```python
from build123d import *

# Parameters (mm, degrees)
F0_R     = 4.35
F1_DEPTH = 2.35
F2_DEPTH = 1
F3_DEPTH = 25


# Not quite as in the source:
# - a feature names something its author has since deleted; it is built from what else it names


with BuildPart() as f1:
    # F0 (on Front) → F1 (new body)
    with BuildSketch(Plane.XZ):
        with BuildLine():
            ThreePointArc((18.9519787885, 1.35), (18.9879909019, 0.6754269088), (19, 0))
            ThreePointArc((19, 0), (18.9879909019, -0.6754269088), (18.9519787885, -1.35))
            ThreePointArc((18.9519787885, -1.35), (13.4350288425, -13.4350288425), (1.35, -18.9519787885))
            ThreePointArc((1.35, -18.9519787885), (0, -19), (-1.35, -18.9519787885))
            ThreePointArc((-1.35, -18.9519787885), (-13.4350288425, -13.4350288425), (-18.9519787885, -1.35))
            ThreePointArc((-18.9519787885, -1.35), (-19, 0), (-18.9519787885, 1.35))
            ThreePointArc((-18.9519787885, 1.35), (-18.0084373125, 6.0577376603), (-15.9148967645, 10.378634832))
            ThreePointArc((-15.9148967645, 10.378634832), (-16.5717114004, 10.7446905008), (-17.1694954771, 11.2008225173))
            ThreePointArc((-17.1694954771, 11.2008225173), (-19.4465872664, 6.4869286792), (-20.4555004828, 1.35))
            ThreePointArc((-20.4555004828, 1.35), (-20.5, 0), (-20.4555004828, -1.35))
            ThreePointArc((-20.4555004828, -1.35), (-14.4956890143, -14.4956890143), (-1.35, -20.4555004828))
            ThreePointArc((-1.35, -20.4555004828), (0, -20.5), (1.35, -20.4555004828))
            ThreePointArc((1.35, -20.4555004828), (14.4956890143, -14.4956890143), (20.4555004828, -1.35))
            ThreePointArc((20.4555004828, -1.35), (20.4888721004, -0.6753666055), (20.5, 0))
            ThreePointArc((20.5, 0), (20.4888721004, 0.6753666055), (20.4555004828, 1.35))
            ThreePointArc((20.4555004828, 1.35), (14.4956890143, 14.4956890143), (1.35, 20.4555004828))
            ThreePointArc((1.35, 20.4555004828), (0, 20.5), (-1.35, 20.4555004828))
            ThreePointArc((-1.35, 20.4555004828), (-5.5075668443, 19.7463087046), (-9.4320097524, 18.2012964382))
            ThreePointArc((-9.4320097524, 18.2012964382), (-9.0377919084, 17.5609883013), (-8.7390902551, 16.8709306653))
            ThreePointArc((-8.7390902551, 16.8709306653), (-5.1507403222, 18.2885175488), (-1.35, 18.9519787885))
            ThreePointArc((-1.35, 18.9519787885), (0, 19), (1.35, 18.9519787885))
            ThreePointArc((1.35, 18.9519787885), (13.4350288425, 13.4350288425), (18.9519787885, 1.35))
        make_face()
        with BuildLine():
            ThreePointArc((-1.35, -18.9519787885), (0, -19), (1.35, -18.9519787885))
            Line((1.35, -18.9519787885), (1.35, -5.7948252778))
            ThreePointArc((1.35, -5.7948252778), (0, -5.95), (-1.35, -5.7948252778))
            Line((-1.35, -5.7948252778), (-1.35, -18.9519787885))
        make_face()
        with BuildLine():
            ThreePointArc((18.9519787885, -1.35), (18.9879909019, -0.6754269088), (19, 0))
            ThreePointArc((19, 0), (18.9879909019, 0.6754269088), (18.9519787885, 1.35))
            Line((18.9519787885, 1.35), (5.7948252778, 1.35))
            ThreePointArc((5.7948252778, 1.35), (5.9110790218, 0.6794444779), (5.95, 0))
            ThreePointArc((5.95, 0), (5.9110790218, -0.6794444779), (5.7948252778, -1.35))
            Line((5.7948252778, -1.35), (18.9519787885, -1.35))
        make_face()
        with BuildLine():
            ThreePointArc((-18.9519787885, 1.35), (-19, 0), (-18.9519787885, -1.35))
            Line((-18.9519787885, -1.35), (-5.7948252778, -1.35))
            ThreePointArc((-5.7948252778, -1.35), (-5.95, 0), (-5.7948252778, 1.35))
            Line((-5.7948252778, 1.35), (-18.9519787885, 1.35))
        make_face()
        with BuildLine():
            Line((1.35, 5.7948252778), (1.35, 18.9519787885))
            ThreePointArc((1.35, 18.9519787885), (0, 19), (-1.35, 18.9519787885))
            Line((-1.35, 18.9519787885), (-1.35, 5.7948252778))
            ThreePointArc((-1.35, 5.7948252778), (0, 5.95), (1.35, 5.7948252778))
        make_face()
        with BuildLine():
            ThreePointArc((5.95, 0), (5.9110790218, 0.6794444779), (5.7948252778, 1.35))
            ThreePointArc((5.7948252778, 1.35), (4.2072853481, 4.2072853481), (1.35, 5.7948252778))
            ThreePointArc((1.35, 5.7948252778), (0, 5.95), (-1.35, 5.7948252778))
            ThreePointArc((-1.35, 5.7948252778), (-4.2072853481, 4.2072853481), (-5.7948252778, 1.35))
            ThreePointArc((-5.7948252778, 1.35), (-5.95, 0), (-5.7948252778, -1.35))
            ThreePointArc((-5.7948252778, -1.35), (-4.2072853481, -4.2072853481), (-1.35, -5.7948252778))
            ThreePointArc((-1.35, -5.7948252778), (0, -5.95), (1.35, -5.7948252778))
            ThreePointArc((1.35, -5.7948252778), (4.2072853481, -4.2072853481), (5.7948252778, -1.35))
            ThreePointArc((5.7948252778, -1.35), (5.9110790218, -0.6794444779), (5.95, 0))
        make_face()
        Circle(F0_R, mode=Mode.SUBTRACT)
    extrude(amount=F1_DEPTH)

    # F0 (on Front) → F2 (join)
    with BuildSketch(Plane.XZ):
        with BuildLine():
            Line((-1.35, 5.7948252778), (-1.35, 18.9519787885))
            ThreePointArc((-1.35, 18.9519787885), (-5.1507403222, 18.2885175488), (-8.7390902551, 16.8709306653))
            ThreePointArc((-8.7390902551, 16.8709306653), (-10.1717962693, 11.2426857548), (-15.9148967645, 10.378634832))
            ThreePointArc((-15.9148967645, 10.378634832), (-18.0084373125, 6.0577376603), (-18.9519787885, 1.35))
            Line((-18.9519787885, 1.35), (-5.7948252778, 1.35))
            ThreePointArc((-5.7948252778, 1.35), (-4.2072853481, 4.2072853481), (-1.35, 5.7948252778))
        make_face()
        with BuildLine():
            ThreePointArc((1.35, -18.9519787885), (13.4350288425, -13.4350288425), (18.9519787885, -1.35))
            Line((18.9519787885, -1.35), (5.7948252778, -1.35))
            ThreePointArc((5.7948252778, -1.35), (4.2072853481, -4.2072853481), (1.35, -5.7948252778))
            Line((1.35, -5.7948252778), (1.35, -18.9519787885))
        make_face()
        with BuildLine():
            Line((5.7948252778, 1.35), (18.9519787885, 1.35))
            ThreePointArc((18.9519787885, 1.35), (13.4350288425, 13.4350288425), (1.35, 18.9519787885))
            Line((1.35, 18.9519787885), (1.35, 5.7948252778))
            ThreePointArc((1.35, 5.7948252778), (4.2072853481, 4.2072853481), (5.7948252778, 1.35))
        make_face()
        with BuildLine():
            ThreePointArc((-18.9519787885, -1.35), (-13.4350288425, -13.4350288425), (-1.35, -18.9519787885))
            Line((-1.35, -18.9519787885), (-1.35, -5.7948252778))
            ThreePointArc((-1.35, -5.7948252778), (-4.2072853481, -4.2072853481), (-5.7948252778, -1.35))
            Line((-5.7948252778, -1.35), (-18.9519787885, -1.35))
        make_face()
        with BuildLine():
            ThreePointArc((-20.4555004828, -1.35), (-20.5, 0), (-20.4555004828, 1.35))
            ThreePointArc((-20.4555004828, 1.35), (-21.8055004828, 0), (-20.4555004828, -1.35))
        make_face()
        with BuildLine():
            ThreePointArc((1.35, -20.4555004828), (0, -20.5), (-1.35, -20.4555004828))
            ThreePointArc((-1.35, -20.4555004828), (0, -21.8055004828), (1.35, -20.4555004828))
        make_face()
        with BuildLine():
            ThreePointArc((20.4555004828, -1.35), (21.8055004828, 0), (20.4555004828, 1.35))
            ThreePointArc((20.4555004828, 1.35), (20.4888721004, 0.6753666055), (20.5, 0))
            ThreePointArc((20.5, 0), (20.4888721004, -0.6753666055), (20.4555004828, -1.35))
        make_face()
        with BuildLine():
            ThreePointArc((1.35, 20.4555004828), (0, 21.8055004828), (-1.35, 20.4555004828))
            ThreePointArc((-1.35, 20.4555004828), (0, 20.5), (1.35, 20.4555004828))
        make_face()
    extrude(amount=F2_DEPTH)

    # F0 (on Front) → F3 (cut)
    with BuildSketch(Plane.XZ):
        with BuildLine():
            ThreePointArc((18.9519787885, 1.35), (18.9879909019, 0.6754269088), (19, 0))
            ThreePointArc((19, 0), (18.9879909019, -0.6754269088), (18.9519787885, -1.35))
            ThreePointArc((18.9519787885, -1.35), (13.4350288425, -13.4350288425), (1.35, -18.9519787885))
            ThreePointArc((1.35, -18.9519787885), (0, -19), (-1.35, -18.9519787885))
            ThreePointArc((-1.35, -18.9519787885), (-13.4350288425, -13.4350288425), (-18.9519787885, -1.35))
            ThreePointArc((-18.9519787885, -1.35), (-19, 0), (-18.9519787885, 1.35))
            ThreePointArc((-18.9519787885, 1.35), (-18.0084373125, 6.0577376603), (-15.9148967645, 10.378634832))
            ThreePointArc((-15.9148967645, 10.378634832), (-16.5717114004, 10.7446905008), (-17.1694954771, 11.2008225173))
            ThreePointArc((-17.1694954771, 11.2008225173), (-19.4465872664, 6.4869286792), (-20.4555004828, 1.35))
            ThreePointArc((-20.4555004828, 1.35), (-20.5, 0), (-20.4555004828, -1.35))
            ThreePointArc((-20.4555004828, -1.35), (-14.4956890143, -14.4956890143), (-1.35, -20.4555004828))
            ThreePointArc((-1.35, -20.4555004828), (0, -20.5), (1.35, -20.4555004828))
            ThreePointArc((1.35, -20.4555004828), (14.4956890143, -14.4956890143), (20.4555004828, -1.35))
            ThreePointArc((20.4555004828, -1.35), (20.4888721004, -0.6753666055), (20.5, 0))
            ThreePointArc((20.5, 0), (20.4888721004, 0.6753666055), (20.4555004828, 1.35))
            ThreePointArc((20.4555004828, 1.35), (14.4956890143, 14.4956890143), (1.35, 20.4555004828))
            ThreePointArc((1.35, 20.4555004828), (0, 20.5), (-1.35, 20.4555004828))
            ThreePointArc((-1.35, 20.4555004828), (-5.5075668443, 19.7463087046), (-9.4320097524, 18.2012964382))
            ThreePointArc((-9.4320097524, 18.2012964382), (-9.0377919084, 17.5609883013), (-8.7390902551, 16.8709306653))
            ThreePointArc((-8.7390902551, 16.8709306653), (-5.1507403222, 18.2885175488), (-1.35, 18.9519787885))
            ThreePointArc((-1.35, 18.9519787885), (0, 19), (1.35, 18.9519787885))
            ThreePointArc((1.35, 18.9519787885), (13.4350288425, 13.4350288425), (18.9519787885, 1.35))
        make_face()
        with BuildLine():
            ThreePointArc((-15.9148967645, 10.378634832), (-12.7472446155, 14.0892780054), (-8.7390902551, 16.8709306653))
            ThreePointArc((-8.7390902551, 16.8709306653), (-9.0377919084, 17.5609883013), (-9.4320097524, 18.2012964382))
            ThreePointArc((-9.4320097524, 18.2012964382), (-13.7536060325, 15.2015894268), (-17.1694954771, 11.2008225173))
            ThreePointArc((-17.1694954771, 11.2008225173), (-16.5717114004, 10.7446905008), (-15.9148967645, 10.378634832))
        make_face()
        with BuildLine():
            ThreePointArc((1.35, 20.4555004828), (0, 21.8055004828), (-1.35, 20.4555004828))
            ThreePointArc((-1.35, 20.4555004828), (0, 20.5), (1.35, 20.4555004828))
        make_face()
        with BuildLine():
            ThreePointArc((-20.4555004828, -1.35), (-20.5, 0), (-20.4555004828, 1.35))
            ThreePointArc((-20.4555004828, 1.35), (-21.8055004828, 0), (-20.4555004828, -1.35))
        make_face()
        with BuildLine():
            ThreePointArc((20.4555004828, -1.35), (21.8055004828, 0), (20.4555004828, 1.35))
            ThreePointArc((20.4555004828, 1.35), (20.4888721004, 0.6753666055), (20.5, 0))
            ThreePointArc((20.5, 0), (20.4888721004, -0.6753666055), (20.4555004828, -1.35))
        make_face()
        with BuildLine():
            ThreePointArc((1.35, -20.4555004828), (0, -20.5), (-1.35, -20.4555004828))
            ThreePointArc((-1.35, -20.4555004828), (0, -21.8055004828), (1.35, -20.4555004828))
        make_face()
    extrude(amount=-F3_DEPTH, mode=Mode.SUBTRACT)


solid = f1.part
```
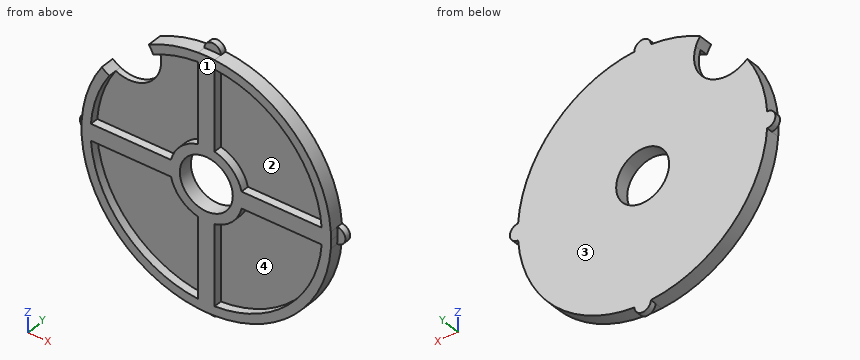
Model file for the job. Use its own axes, mm. Face numbers are marked on the shaded views. A direction names the side the tool comes from. Give positions to 0.01 mm unless a question says otherwise; leave off trailing zeros. Order: outer loops, then holes, each group sorted by start corner. A loop starts at its lowest first (then second) coordinate and runs counter-clockwise, first axis right, second up.
1) Saw through at B-B, the plane y = -0.45. Write the cut outline in (x, z).
2) 3-axis set-ups, long thin cutter, end or side, ignore diameter. For the marked faces 3 and 4: which of +Z, -Z, +X, -X, +Y, -Y reach the whole face in a straight line?
3) Mould opens along Z. For the marked faces 1 and 2 say: +Z half, -Z half, draft (parallel to the pull), parting line (faces both ways), or undercut.
4) Saw through at C-C, the plane z = -3. Write the cut outline in (x, y), then the cut area to 3 significant figures.
5) Saw through at D-D, the plane x = 13. Write the cut outline in (y, z), then the cut area to 3 significant figures.
6) Wall check: probe 1 along Z at (x, y) = (0, -1.55); probe 2 along Z at (x, y) = (0, -0.85); probe 3 along Z at (x, y) = (-7.5, -1.05). Give the ranges that are in metal, low to high.
7) Saw through at A-A, the plane x = 0. Write the cut outline in (y, z).
8) Pin check, flat tips, straight feed: pin 1 (5 mm diameter, centred on x = 6, z = -10.5, fed in from +Y); pin 2 (1 mm diameter, centred on y = -1, z = -7.5, fed in from -X); pin 3 (1.1 mm diameter, centred on x = -11.5, y = -1.5, fed in from -Z); pin 4 (1.1 mm diameter, centred on x = 9.5, y = -1.5, fed in from +Z). Stop position of each tip, or through.
Computed:
1. outline: (-20.46, -1.35) arc R20.5 ccw to (-1.35, -20.46) arc R1.35 ccw to (1.35, -20.46) arc R20.5 ccw to (20.46, -1.35) arc R1.35 ccw to (20.46, 1.35) arc R20.5 ccw to (1.35, 20.46) arc R1.35 ccw to (-1.35, 20.46) arc R20.5 ccw to (-9.43, 18.2) arc R5.25 cw to (-17.17, 11.2) arc R20.5 ccw to (-20.46, 1.35) arc R1.35 ccw to start; hole circle Ø8.7 at (0, 0)
2. face 3: +Z, -Z, +X, -X, +Y
2. face 4: -Y
3. face 1: draft
3. face 2: undercut
4. outline: (-20.28, -2.35) - (-18.76, -2.35) - (-18.76, -1) - (-5.14, -1) - (-5.14, -2.35) - (-3.15, -2.35) - (-3.15, 0) - (-20.28, 0) - close; (3.15, -2.35) - (5.14, -2.35) - (5.14, -1) - (18.76, -1) - (18.76, -2.35) - (20.28, -2.35) - (20.28, 0) - (3.15, 0) - close
4. area: 43.7 mm2
5. outline: (-2.35, -15.85) - (0, -15.85) - (0, 15.85) - (-2.35, 15.85) - (-2.35, 13.86) - (-1, 13.86) - (-1, 1.35) - (-2.35, 1.35) - (-2.35, -1.35) - (-1, -1.35) - (-1, -13.86) - (-2.35, -13.86) - close
5. area: 40.7 mm2
6. probe 1: z = -20.5 to -4.35, 4.35 to 20.5
6. probe 2: z = -21.81 to -4.35, 4.35 to 21.81
6. probe 3: z = -19.08 to -17.46, -1.35 to 1.35, 17.46 to 19.08
7. outline: (-2.35, -20.5) - (-1, -20.5) - (-1, -21.81) - (0, -21.81) - (0, -4.35) - (-2.35, -4.35) - close; (-2.35, 4.35) - (0, 4.35) - (0, 21.81) - (-1, 21.81) - (-1, 20.5) - (-2.35, 20.5) - close
8. pin 1: stops at y = 0
8. pin 2: stops at x = -19.27
8. pin 3: stops at z = -17.33
8. pin 4: stops at z = 18.44
